```python
from build123d import *

# Parameters (mm, degrees)
SKETCH_1_R          = 3.5
SKETCH_1_R_2        = 2
EXTRUDE_397_DEPTH   = 4
SKETCH_1_3_R        = 2
EXTRUDE_432_DEPTH   = 35
CUT_EXTRUDE_1_DEPTH = 2


with BuildPart() as part:
    # Sketch 1 → Extrude 397 (new body)
    with BuildSketch(Plane(origin=(0, 0, 0), x_dir=(1, 0, 0), z_dir=(0, 1, 0))):
        with Locations(Location((0, 0, 0), (0, 0, 270))):
            Circle(SKETCH_1_R)
        Circle(SKETCH_1_R_2, mode=Mode.SUBTRACT)
        Circle(SKETCH_1_R_2)
    extrude(amount=EXTRUDE_397_DEPTH)

    # Sketch 1_3 → Extrude 432 (add)
    with BuildSketch(Plane(origin=(0, 0, 0), x_dir=(1, 0, 0), z_dir=(0, 1, 0))):
        with Locations(Location((0, 0, 0), (0, 0, 270))):
            Circle(SKETCH_1_3_R)
    extrude(amount=-EXTRUDE_432_DEPTH)

    # Sketch 2 → Cut-Extrude 1 (cut)
    with BuildSketch(Plane(origin=(0, 4, 0), x_dir=(1, 0, 0), z_dir=(0, 1, 0))):
        Polygon((1.732050808, 0), (0.866025404, 1.5), (-0.866025404, 1.5), (-1.732050808, 0), (-0.866025404, -1.5), (0.866025404, -1.5), align=None)
    extrude(amount=-CUT_EXTRUDE_1_DEPTH, mode=Mode.SUBTRACT)


solid = part.part
```
For this review, take the finished solid that the model builds, in its own axes (mm). A direction names the side the tool comes from. Give positions to 0.01 mm unless a question says otherwise; leave off trailing zeros. Write each loop counter-clockwise with the first axis right and the second up, starting at its lowest first coordinate (ties: lowest second). Pieces come first, ordered by that corner, then holes.
Item 1: Machinability: for faces 1 (the face through (-2, 0, 2)), 2 (the face through (1.293, 3.014, 0.76)), 3 (the face through (-3.417, 1.972, -0.759)), which of the approach directions +Z, -Z, +X, -X, +Y, -Y give a long, thin tool a straight path to every point of the face, cutting with its end or side? Answer none if there is none.
Item 2: Wall thickness on probe 1 along Y at (x, z) = (1.5, -2.75); probe 2 along Z at (x, y) = (1, -32.5): over which ranges is each line inside the solid? List them lowest first.
Item 3: Take a section at A-A (x = 0). Give the boundary of the cut face in (y, z), and give its area (3 significant figures).
Item 4: Insertion check: P1, Ø3, axis at x = -0.5, y = -18, coming from the -Z side; P2, Ø4, axis at y = -25, z = 1, coming from the -X side; P3, Ø1.5, axis at x = -1, y = -1, coming from the +Z side. Each pin has a flat end and moves straight along its axis. Give the tip position at first contact, or say it passes through.
Item 5: Take a section at D-D (z = 3). Give the boundary of the cut face in (x, y), and give its area (3 significant figures).
Item 6: Take a section at C-C (z = 0.5). Give the boundary of the cut face in (x, y).
Item 7: Take a section at B-B (y = -16.5). Give the boundary of the cut face in (x, z), and give its area (3 significant figures).
Item 8: The part is to be moulded in two halves that separate along Z. For faces 4 (the face through (0, 4, 2)), 5 (the face through (-1.305, 3.014, 0.74)), 6 (the face through (-2, -17, 0)), say which applies: +Z half, -Z half, draft (parallel to the pull), parting line (faces both ways), or undercut.
Established:
1. face 1: -Y
1. face 2: +Y
1. face 3: +Y, -Y
2. probe 1: y = 0 to 4
2. probe 2: z = -1.73 to 1.73
3. outline: (-35, -2) - (0, -2) - (0, -3.5) - (4, -3.5) - (4, -1.5) - (2, -1.5) - (2, 1.5) - (4, 1.5) - (4, 3.5) - (0, 3.5) - (0, 2) - (-35, 2) - close
3. area: 162 mm2
4. P1: stops at z = -2
4. P2: stops at x = -2
4. P3: stops at z = 1.98
5. outline: (-1.8, 0) - (1.8, 0) - (1.8, 4) - (-1.8, 4) - close
5. area: 14.4 mm2
6. outline: (-3.46, 0) - (-1.94, 0) - (-1.94, -35) - (1.94, -35) - (1.94, 0) - (3.46, 0) - (3.46, 4) - (1.44, 4) - (1.44, 2) - (-1.44, 2) - (-1.44, 4) - (-3.46, 4) - close
7. outline: circle Ø4 at (0, 0)
7. area: 12.6 mm2
8. face 4: draft
8. face 5: undercut
8. face 6: parting line
